```python
from build123d import *

# Parameters (mm, degrees)
SKETCH1_W           = 43
SKETCH1_H           = 43
SKETCH1_W_2         = 41
SKETCH1_H_2         = 39
BOSS_EXTRUDE1_DEPTH = 18
SKETCH2_W           = 43
SKETCH2_H           = 43
BOSS_EXTRUDE2_DEPTH = 0.8
SKETCH3_R           = 0.75
CUT_EXTRUDE1_DEPTH  = 10.8
BOSS_EXTRUDE3_START = 4
SKETCH4_R           = 2.55
SKETCH4_R_2         = 0.75
BOSS_EXTRUDE3_DEPTH = 4
CUT_EXTRUDE2_DEPTH  = 4


with BuildPart() as part:
    # Sketch1 → Boss-Extrude1 (new body)
    with BuildSketch(Plane(origin=(0, 0, 0), x_dir=(1, 0, 0), z_dir=(0, 1, 0))):
        Rectangle(SKETCH1_W, SKETCH1_H)
        Rectangle(SKETCH1_W_2, SKETCH1_H_2, mode=Mode.SUBTRACT)
    extrude(amount=BOSS_EXTRUDE1_DEPTH)

    # Sketch2 → Boss-Extrude2 (add)
    with BuildSketch(Plane.XZ):
        Rectangle(SKETCH2_W, SKETCH2_H)
    extrude(amount=BOSS_EXTRUDE2_DEPTH)

    # Sketch3 → Cut-Extrude1 (cut)
    with BuildSketch(Plane(origin=(0, 0, 0), x_dir=(1, 0, 0), z_dir=(0, 1, 0))):
        with Locations(Location((18.3, 17.3, 0), (0, 0, 270))):
            Circle(SKETCH3_R)
        with Locations(Location((-18.3, 17.3, 0), (0, 0, 270))):
            Circle(SKETCH3_R)
        with Locations(Location((-18.3, -17.3, 0), (0, 0, 270))):
            Circle(SKETCH3_R)
        with Locations(Location((18.3, -17.3, 0), (0, 0, 270))):
            Circle(SKETCH3_R)
    extrude(amount=-CUT_EXTRUDE1_DEPTH, mode=Mode.SUBTRACT)

    # Sketch4 → Boss-Extrude3 (add)
    # profile 1 of 4: a face of its own
    with BuildSketch(Plane(origin=(0, 0, 0), x_dir=(1, 0, 0), z_dir=(0, 1, 0)).offset(BOSS_EXTRUDE3_START)):
        with Locations((-18.3, 17.3)):
            Circle(SKETCH4_R)
        with Locations(Location((-18.3, 17.3, 0), (0, 0, 270))):
            Circle(SKETCH4_R_2, mode=Mode.SUBTRACT)
    # profile 2 of 4: a face of its own
    with BuildSketch(Plane(origin=(0, 0, 0), x_dir=(1, 0, 0), z_dir=(0, 1, 0)).offset(BOSS_EXTRUDE3_START)):
        with Locations((18.3, 17.3)):
            Circle(SKETCH4_R)
        with Locations(Location((18.3, 17.3, 0), (0, 0, 270))):
            Circle(SKETCH4_R_2, mode=Mode.SUBTRACT)
    # profile 3 of 4: a face of its own
    with BuildSketch(Plane(origin=(0, 0, 0), x_dir=(1, 0, 0), z_dir=(0, 1, 0)).offset(BOSS_EXTRUDE3_START)):
        with Locations((18.3, -17.3)):
            Circle(SKETCH4_R)
        with Locations(Location((18.3, -17.3, 0), (0, 0, 270))):
            Circle(SKETCH4_R_2, mode=Mode.SUBTRACT)
    # profile 4 of 4: a face of its own
    with BuildSketch(Plane(origin=(0, 0, 0), x_dir=(1, 0, 0), z_dir=(0, 1, 0)).offset(BOSS_EXTRUDE3_START)):
        with Locations((-18.3, -17.3)):
            Circle(SKETCH4_R)
        with Locations(Location((-18.3, -17.3, 0), (0, 0, 270))):
            Circle(SKETCH4_R_2, mode=Mode.SUBTRACT)
    extrude(amount=-BOSS_EXTRUDE3_DEPTH)

    # Sketch5 → Cut-Extrude2 (cut)
    with BuildSketch(Plane(origin=(21.5, 0, 0), x_dir=(0, 0, -1), z_dir=(1, 0, 0))):
        with BuildLine():
            Line((-12.25, 12), (-12.25, 18))
            Line((-12.25, 18), (-6.75, 18))
            Line((-6.75, 18), (-6.75, 12))
            ThreePointArc((-6.75, 12), (-9.5, 9.25), (-12.25, 12))
        make_face()
    extrude(amount=-CUT_EXTRUDE2_DEPTH, mode=Mode.SUBTRACT)


solid = part.part
```
Part model, mm, in its own coordinate system. A direction names the side the tool comes from. Coordinates: 2 decimals unless noted, no trailing zeros. Write each loop counter-clockwise with the first axis right and the second up, starting at its lowest first coordinate (ties: lowest second). Pieces come first, ordered by that corner, then holes.
Item 1: Slice it at B-B (x = -18.3). Write the cut outline in (y, z).
Item 2: Mould opens along Z. For faces 1 (the face through (0, 9, -21.5)), 2 (the face through (16.451, 2.028, -15.544)), 3 (the face through (0, 9, 21.5)) say: released by +Z, released by -Z, zero draft, split by the parting line, or undercut.
Item 3: Which spindle directions (+Z, -Z, +X, -X, +Y, -Y) get a long thin tool onto all of the face, cutting with end or side? Do faces 4 (the face through (21, 15, 12.25)), 5 (the face through (0, -0.8, 0)), 6 (the face through (17.6, 4, 16.6)). Say none if no direction does.
Item 4: Pin check, flat tips, straight feed: pin 1 (2 mm diameter, centred on x = 18.3, z = -17.3, fed in from +Y); pin 2 (0.9 mm diameter, centred on x = 18.3, z = 17.3, fed in from -Y); pin 3 (6 mm diameter, centred on x = -7.5, z = 2, fed in from +Y). Stop position of each tip, or through.
Item 5: Slice it at A-A (y = 6). Write the cut outline in (x, z), and give its area (3 significant figures).
Item 6: Slice it at D-D (z = 1). Write the cut outline in (x, y).
Item 7: Slice it at C-C (z = -17.3). Write the cut outline in (x, y).
Item 8: Probe line 1 (X direction, y = 1.1, z = 17.3); line 2 (Z direction, x = 7, y = 12.5); line 3 (X direction, y = 0.75, z = 8). List the from-to ranges inside material, lowest first.
Results found:
1. outline: (-0.8, -21.5) - (18, -21.5) - (18, -19.5) - (4, -19.5) - (4, -18.05) - (-0.8, -18.05) - close; (-0.8, -16.55) - (4, -16.55) - (4, -14.75) - (0, -14.75) - (0, 14.75) - (4, 14.75) - (4, 16.55) - (-0.8, 16.55) - close; (-0.8, 18.05) - (4, 18.05) - (4, 19.5) - (18, 19.5) - (18, 21.5) - (-0.8, 21.5) - close
2. face 1: released by -Z
2. face 2: undercut
2. face 3: released by +Z
3. face 4: +X, +Y
3. face 5: +Z, -Z, +X, -X, -Y
3. face 6: +Y
4. pin 1: stops at y = 4
4. pin 2: passes through
4. pin 3: stops at y = 0
5. outline: (-21.5, -21.5) - (21.5, -21.5) - (21.5, 21.5) - (-21.5, 21.5) - close; hole (-20.5, -19.5) - (20.5, -19.5) - (20.5, 19.5) - (-20.5, 19.5) - close
5. area: 250 mm2
6. outline: (-21.5, -0.8) - (21.5, -0.8) - (21.5, 18) - (20.5, 18) - (20.5, 0) - (-20.5, 0) - (-20.5, 18) - (-21.5, 18) - close
7. outline: (-21.5, -0.8) - (-19.05, -0.8) - (-19.05, 4) - (-20.5, 4) - (-20.5, 18) - (-21.5, 18) - close; (-17.55, -0.8) - (17.55, -0.8) - (17.55, 4) - (15.75, 4) - (15.75, 0) - (-15.75, 0) - (-15.75, 4) - (-17.55, 4) - close; (19.05, -0.8) - (21.5, -0.8) - (21.5, 18) - (20.5, 18) - (20.5, 4) - (19.05, 4) - close
8. line 1: x = -21.5 to -19.05, -17.55 to -15.75, 15.75 to 17.55, 19.05 to 21.5
8. line 2: z = -21.5 to -19.5, 19.5 to 21.5
8. line 3: x = -21.5 to -20.5, 20.5 to 21.5
